Input: part model. Units: mm. Frame: model coordinates. A direction names the side the tool comes from. Coordinates: 2 decimals unless noted, no trailing zeros. Loops run counter-clockwise (first coordinate to the right, second up) from the corner with the lowest first, then second, coordinate; pieces in that order, holes last. Notation, with made-up numbers: M -7.75,2 L -3.75,2 A24 ccw -3.75,15 Z; hole C -33.5,83.5 d7. An arc over 180 degrees is marked long. Use a Markdown table: item, result. Add a question column.
1. Line query: L1, parallel to Z at x = 4, y = 3.5; L2, parallel to X at y = -1.15, z = -5; L3, parallel to Y at x = 2, z = -1. Output: solid intervals per line, ascending. Write a range as [from, to].
2. Section D-D on y = -1.5. Output: boundary loops of the cut face in (x, z).
3. Pin query (flat end, axial travel): pin 1 (4 mm diameter, centred on y = 6.5, z = -8, fed in from +X); pin 2 (3 mm diameter, centred on x = 1, z = -6.5, fed in from +Y). Return the tip coordinate at first contact, or that it passes through.
4. Section C-C on x = 4.75. Output: boundary loops of the cut face in (y, z).
5. Set-up query: faces 1 (the flat face through (4, 3, -8)), 2 (the flat face through (6, -1.6, -4.9)). Return all of +Z, -Z, +X, -X, +Y, -Y with unobstructed straight access to the full face (end or side cutting, diameter ignored); none if empty.
6. Section B-B on y = 5.25. Output: boundary loops of the cut face in (x, z).
7. Section A-A on z = -5. Output: boundary loops of the cut face in (x, y), then the cut area to 3 significant figures.
8. Draft query along Z for faces 3 (the flat face through (2, 3, -5)), 4 (the flat face through (2, 2, 0)), 5 (the flat face through (0, 3, -5)). Return one class per face: +Z half, -Z half, draft (parallel to the pull), parting line (faces both ways), or undercut.
```python
from build123d import *

# Parameters (mm, degrees)
CROQUIS1_W              = 4
CROQUIS1_H              = 6
CROQUIS1_R              = 1
SALIENTE_EXTRUIR1_DEPTH = 2
SALIENTE_EXTRUIR2_DEPTH = 8
CROQUIS2_R              = 1
CORTAR_EXTRUIR1_DEPTH   = 14.416407865
REDONDEO1_R             = 10


with BuildPart() as part:
    # Croquis1 → Saliente-Extruir1 (new body)
    # profile 1 of 2: a face of its own
    with BuildSketch(Plane(origin=(0, 0, 0), x_dir=(1, 0, 0), z_dir=(0, 1, 0))):
        with Locations((4, 5)):
            Rectangle(CROQUIS1_W, CROQUIS1_H)
        with Locations(Location((4, 5, 0), (0, 0, 270))):
            Circle(CROQUIS1_R, mode=Mode.SUBTRACT)
    # profile 2 of 2: a face of its own
    with BuildSketch(Plane(origin=(0, 0, 0), x_dir=(1, 0, 0), z_dir=(0, 1, 0))):
        Polygon((6, 0), (6, 2), (2, 2), (2, 8), (6, 8), (6, 10), (0, 10), (0, 0), align=None)
    extrude(amount=-SALIENTE_EXTRUIR1_DEPTH)

    # Croquis1<3> → Saliente-Extruir2 (add)
    with BuildSketch(Plane(origin=(0, 0, 0), x_dir=(1, 0, 0), z_dir=(0, 1, 0))):
        Polygon((6, 0), (6, 2), (2, 2), (2, 8), (6, 8), (6, 10), (0, 10), (0, 0), align=None)
    extrude(amount=SALIENTE_EXTRUIR2_DEPTH)

    # Croquis2 → Cortar-Extruir1 (cut, through all)
    with BuildSketch(Plane(origin=(2, 0, 0), x_dir=(0, 0, -1), z_dir=(1, 0, 0))):
        with Locations((5, 5.5)):
            Circle(CROQUIS2_R)
    extrude(amount=-CORTAR_EXTRUIR1_DEPTH, mode=Mode.SUBTRACT)

    # Redondeo1
    # the kernel refuses this fillet: 10 mm, written as the material it takes off along each edge
    with BuildSketch(Plane(origin=(6, 8, 22.912878475), x_dir=(0, -1, 0), z_dir=(0, 0, -1))) as redondeo1_piece_1:
        with BuildLine():
            CenterArc((9.16515139, 10), REDONDEO1_R, 203.578178478, 66.421821522)
            Line((0, 6), (-0.183303028, 5.92))
            ThreePointArc((-0.183303028, 5.92), (-0.2, 3), (-0.2, 0))
            Line((-0.2, 0), (0, -0.2))
            Line((0, -0.2), (9.16515139, -0.2))
            Line((9.16515139, -0.2), (9.16515139, 0))
        make_face()
    extrude(amount=47.82575695, mode=Mode.SUBTRACT)


solid = part.part
```
Answers below:
| question | item | result |
|---|---|---|
| 1 | L1 | z = [-10, -8], [-2, 0] |
| 1 | L2 | x = [0, 3], [5, 6] |
| 1 | L3 | y = [-2, 6.83] |
| 2 | outline | M 0,-10 L 6,-10 L 6,0 L 0,0 Z; hole C 4,-5 d2 |
| 3 | pin 1 | stops at x = 4.24 |
| 3 | pin 2 | stops at y = 8 |
| 4 | outline | M -2,-10 L 3.68,-10 L 3.68,-8 L 0,-8 L 0,-5.66 L -2,-5.66 Z; M -2,-4.34 L 0,-4.34 L 0,-2 L 3.68,-2 L 3.68,0 L -2,0 Z |
| 5 | face 1 | +X, +Y |
| 5 | face 2 | +Z, -Z, +X, +Y, -Y |
| 6 | outline | M 0,-10 L 3.67,-10 L 3.67,-8 L 2,-8 L 2,-5.97 L 0,-5.97 Z; M 0,-4.03 L 2,-4.03 L 2,-2 L 3.67,-2 L 3.67,0 L 0,0 Z |
| 7 | outline | M 0,-2 L 3,-2 L 3,0 L 2,0 L 2,4.5 L 0,4.5 Z; M 0,6.5 L 2,6.5 L 2,6.83 A10 ccw 0,8 Z; M 5,-2 L 6,-2 L 6,-1.17 A10 ccw 5.93,0 L 5,0 Z |
| 7 | area | 18.9 mm² |
| 8 | face 3 | undercut |
| 8 | face 4 | +Z half |
| 8 | face 5 | draft |
